Verification items for the finished model (mm, model axes). Face numbers are marked on the shaded views. A direction names the side the tool comes from. Coordinates: 2 decimals unless noted, no trailing zeros. Write each loop counter-clockwise with the first axis right and the second up, starting at its lowest first coordinate (ties: lowest second). Pieces come first, ordered by that corner, then holes. Notation, with made-up numbers: M 67,60 L 123,60 A15 cw 123,83 Z; hole C 37,20.5 d1. An arc over 180 degrees is marked long. Answer in a Markdown table with one row per item.
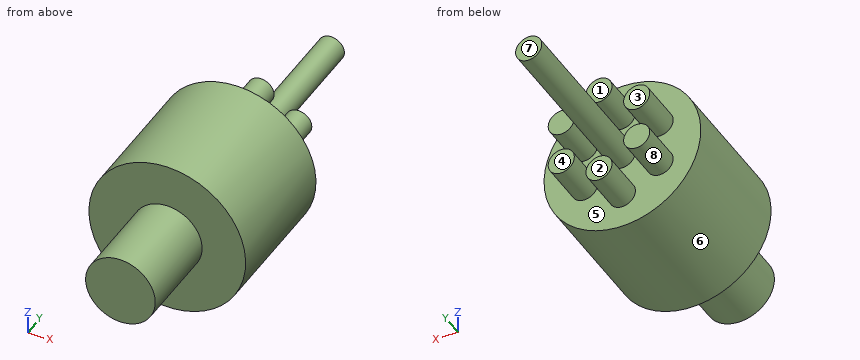
from build123d import *

# Parameters (mm, degrees)
SKETCH2_R           = 3
BOSS_EXTRUDE1_DEPTH = 10
CIRPATTERN1_COUNT   = 6


with BuildPart() as part:
    # Sketch1 → Revolve1 (revolve)
    with BuildSketch(Plane(origin=(0, 0, 0), x_dir=(0, 0, -1), z_dir=(1, 0, 0))):
        Polygon((0, 0), (-8, 0), (-8, 20), (-18, 20), (-18, 50), (-3, 50), (-3, 90), (0, 90), align=None)
    revolve(axis=Axis((0, 90, 0), (0, -1, 0)))

    # Sketch2 → Boss-Extrude1 (add)
    with BuildSketch(Plane(origin=(0, 50, 0), x_dir=(1, 0, 0), z_dir=(0, 1, 0))):
        with Locations((0, 10)):
            Circle(SKETCH2_R)
    boss_extrude1 = extrude(amount=BOSS_EXTRUDE1_DEPTH)

    # CirPattern1: Boss-Extrude1 ×6 about axis
    cirpattern1_axis = Axis((0, 0, 0), (0, 1, 0))
    for i in range(1, CIRPATTERN1_COUNT):
        add(boss_extrude1.rotate(cirpattern1_axis, i * 360 / CIRPATTERN1_COUNT))


solid = part.part
1) Sectioned sample at A-A (x = 0). Record the cut outline in (y, z), then the cut area to 3 significant figures.
Response values:
| item | result |
|---|---|
| outline | M 0,-8 L 20,-8 L 20,-18 L 50,-18 L 50,-13 L 60,-13 L 60,-7 L 50,-7 L 50,-3 L 90,-3 L 90,3 L 50,3 L 50,7 L 60,7 L 60,13 L 50,13 L 50,18 L 20,18 L 20,8 L 0,8 Z |
| area | 1,760 mm² |
2) Release check for a two-part mould opening along X. For the marked faces 6, 7 and 8 record: +X half, -X half, draft (parallel to the pull), parting line (faces both ways), or undercut.
Response values:
| item | result |
|---|---|
| face 6 | parting line |
| face 7 | draft |
| face 8 | undercut |
3) Sectioned sample at B-B (z = 0). Record the cut outline in (x, y), then the cut area to 3 significant figures.
Response values:
| item | result |
|---|---|
| outline | M -18,20 L -8,20 L -8,0 L 8,0 L 8,20 L 18,20 L 18,50 L 3,50 L 3,90 L -3,90 L -3,50 L -18,50 Z |
| area | 1,640 mm² |
4) Depth check by flat-ended pin: pin 1 (5 mm diameter, centred on x = 1, z = -10, fed in from +Y); pin 2 (2 mm diameter, centred on x = 7, y = 30, fed in from +Z); pin 3 (4 mm diameter, centred on x = 12.5, y = 32.5, fed in from +Z); pin 4 (1 mm diameter, centred on x = 4, y = 53, fed in from +Z). Enter the tip coordinate at first touch or a pass-through.
Response values:
| item | result |
|---|---|
| pin 1 | stops at y = 60 |
| pin 2 | stops at z = 16.97 |
| pin 3 | stops at z = 14.62 |
| pin 4 | passes through |
5) Tool access check on the marked faces 1, 2, 3, 4 and 5. Record the directions out of +Z, -Z, +X, -X, +Y, -Y that give a thin tool (end or side, any length) a straight path to the whole face; none if there is none.
Response values:
| item | result |
|---|---|
| face 1 | +Z, +X, -X, +Y |
| face 2 | -Z, +X, -X, +Y |
| face 3 | +Z, -Z, -X, +Y |
| face 4 | +Z, -Z, +X, +Y |
| face 5 | +Y |
6) Sectioned sample at C-C (y = 35.5). Record the cut outline in (x, z).
Response values:
| item | result |
|---|---|
| outline | C 0,0 d36 |
7) Thickness scan on L1, parallel to Z at x = -9, y = 55; L2, parallel to Y at x = 10, z = 4.5; L3, parallel to Y at x = -4.5, z = -5. Record the ranges inside material, lowest first. Write a range as [from, to].
Response values:
| item | result |
|---|---|
| L1 | z = [-7.98, -2.02], [2.02, 7.98] |
| L2 | y = [20, 60] |
| L3 | y = [0, 50] |
8) Sectioned sample at D-D (z = -4.5). Record the cut outline in (x, y).
Response values:
| item | result |
|---|---|
| outline | M -17.43,20 L -6.61,20 L -6.61,0 L 6.61,0 L 6.61,20 L 17.43,20 L 17.43,50 L 11.62,50 L 11.62,60 L 5.7,60 L 5.7,50 L -5.7,50 L -5.7,60 L -11.62,60 L -11.62,50 L -17.43,50 Z |
